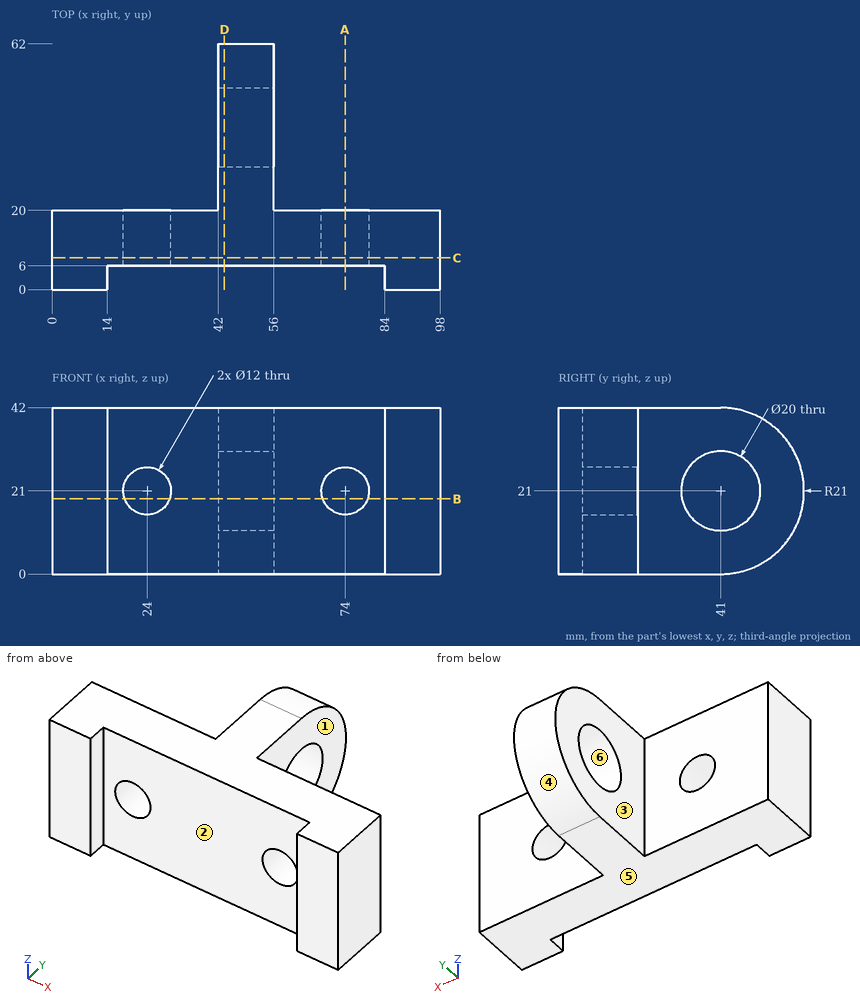
Source: three-view drawing plus pictorial views. Frame: mm from the lowest corner of the part. A direction names the side the tool comes from. Give positions to 0.01 mm unless a question says otherwise; leave off trailing zeros. Write each loop counter-clockwise with the first axis right and the second up, starting at its lowest first coordinate (ties: lowest second). Pieces come first, ordered by that corner, then holes. Notation, with made-up numbers: (81.25, 76.5) -> (134.25, 76.5) arc R18 cw to (134.25, 98.5) -> close; hole circle Ø6 at (46.5, 71.5). An arc over 180 degrees is marked (long way). Answer in a Markdown table with one row per item.
(1) Section query C-C on y = 8. Return loops of the section in (x, z).
Answers below:
| item | result |
|---|---|
| outline | (0, 0) -> (98, 0) -> (98, 42) -> (0, 42) -> close; hole circle Ø12 at (24, 21); hole circle Ø12 at (74, 21) |
(2) Section query B-B on z = 19. Return loops of the section in (x, y), then the cut area to 3 significant figures.
Answers below:
| item | result |
|---|---|
| outline | (0, 0) -> (14, 0) -> (14, 6) -> (18.34, 6) -> (18.34, 20) -> (0, 20) -> close; (29.66, 6) -> (68.34, 6) -> (68.34, 20) -> (56, 20) -> (56, 31.2) -> (42, 31.2) -> (42, 20) -> (29.66, 20) -> close; (42, 50.8) -> (56, 50.8) -> (56, 61.9) -> (42, 61.9) -> close; (79.66, 6) -> (84, 6) -> (84, 0) -> (98, 0) -> (98, 20) -> (79.66, 20) -> close |
| area | 1,540 mm^2 |
(3) Ray query, line 1 along X through (y, z) = (14.75, 21); line 2 along Y through (x, z) = (47.25, 21); line 3 along Y through (x, z) = (62, 34). Return the intervals inside material, ascending. Write a range as [from, to].
Answers below:
| item | result |
|---|---|
| line 1 | [0, 18], [30, 68], [80, 98] |
| line 2 | [6, 31], [51, 62] |
| line 3 | [6, 20] |
(4) Draft query along Z for the marked faces 4, 5 and 6. Return one class per face: +Z half, -Z half, draft (parallel to the pull), parting line (faces both ways), or undercut.
Answers below:
| item | result |
|---|---|
| face 4 | parting line |
| face 5 | -Z half |
| face 6 | undercut |
(5) Section query A-A on x = 74. Return loops of the section in (y, z), then the cut area to 3 significant figures.
Answers below:
| item | result |
|---|---|
| outline | (6, 0) -> (20, 0) -> (20, 15) -> (6, 15) -> close; (6, 27) -> (20, 27) -> (20, 42) -> (6, 42) -> close |
| area | 420 mm^2 |
(6) Set-up query: the marked faces 1, 2 and 3. Return all of +Z, -Z, +X, -X, +Y, -Y with unobstructed straight access to the full face (end or side cutting, diameter ignored); none if empty.
Answers below:
| item | result |
|---|---|
| face 1 | +Z, -Z, +X, +Y |
| face 2 | +Z, -Z, -Y |
| face 3 | +Z, -Z, -X, +Y |
(7) Section query D-D on x = 43.5. Return loops of the section in (y, z), then the cut area to 3 significant figures.
Answers below:
| item | result |
|---|---|
| outline | (6, 0) -> (41, 0) arc R21 ccw to (41, 42) -> (6, 42) -> close; hole circle Ø20 at (41, 21) |
| area | 1,850 mm^2 |
(8) Pin query (flat end, axial travel): pin 1 (3 mm diameter, centred on y = 3.5, z = 26.5, fed in from -X); pin 2 (1 mm diameter, centred on x = 69.5, z = 10, fed in from -Y); pin 3 (1.5 mm diameter, centred on y = 27.5, z = 16, fed in from +X); pin 4 (21 mm diameter, centred on x = 73.5, z = 22.5, fed in from +Y). Return the tip coordinate at first contact, or that it passes through.
Answers below:
| item | result |
|---|---|
| pin 1 | x = 0 |
| pin 2 | y = 6 |
| pin 3 | x = 56 |
| pin 4 | y = 20 |
